The listing builds one solid part. Answer for the finished solid, in the listing's coordinates (mm). Face numbers are marked on the shaded views. A direction names the side the tool comes from. Round coordinates to 2 decimals unless told otherwise and drop trailing zeros. Loops run counter-clockwise (first coordinate to the right, second up) from the corner with the lowest first, then second, coordinate; pieces in that order, holes last. Notation, with made-up numbers: (61.5, -23) -> (101.5, -23) arc R21 ccw to (101.5, -15) -> close; hole circle Ø11 at (11, 4). An arc over 180 degrees is marked (long way). One line per question, with ' | ' between items.
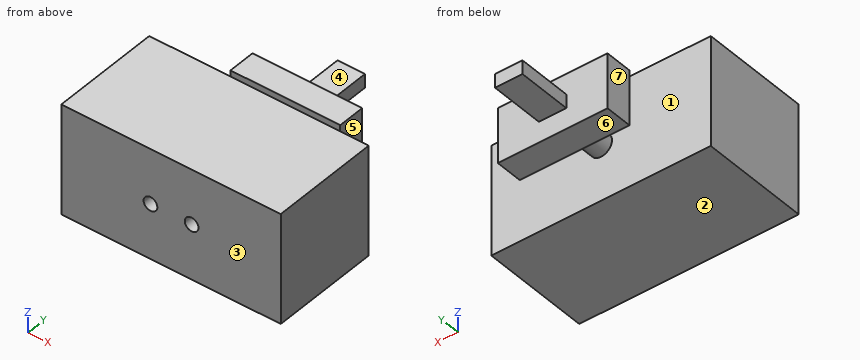
from build123d import *

# Parameters (mm, degrees)
F0_W     = 50.8
F0_H     = 25.4
F0_R     = 1.5875
F1_DEPTH = 25.4
F2_R     = 2.54
F3_DEPTH = 7.62
F4_W     = 25.4
F4_H     = 12.7
F5_DEPTH = 6.35
F6_W     = 6.35
F6_H     = 3.175
F7_DEPTH = 12.7
F8_DEPTH = 19.05


with BuildPart() as f1:
    # F0 (on Front) → F1 (new body)
    with BuildSketch(Plane.XZ):
        Rectangle(F0_W, F0_H)
        with Locations((-4.7625, 0)):
            Circle(F0_R, mode=Mode.SUBTRACT)
        with Locations((4.7625, 0)):
            Circle(F0_R, mode=Mode.SUBTRACT)
        with Locations((4.7625, 0)):
            Circle(F0_R)
        with Locations((-4.7625, 0)):
            Circle(F0_R)
    extrude(amount=-F1_DEPTH)

    # F2 (on face) → F3 (join)
    with BuildSketch(Plane(origin=(0, 25.4, 0), x_dir=(-1, 0, 0), z_dir=(0, 1, 0))):
        Circle(F2_R)
    extrude(amount=F3_DEPTH)

    # F4 (on face) → F5 (join)
    with BuildSketch(Plane(origin=(0, 33.02, 0), x_dir=(-1, 0, 0), z_dir=(0, 1, 0))):
        Rectangle(F4_W, F4_H)
    extrude(amount=F5_DEPTH)

    # F6 (on face) → F7 (join)
    with BuildSketch(Plane(origin=(0, 39.37, 0), x_dir=(-1, 0, 0), z_dir=(0, 1, 0))):
        Rectangle(F6_W, F6_H)
    extrude(amount=F7_DEPTH)

    # F0 (on Front) → F8 (cut)
    with BuildSketch(Plane.XZ):
        with Locations((4.7625, 0)):
            Circle(F0_R)
        with Locations((-4.7625, 0)):
            Circle(F0_R)
    extrude(amount=-F8_DEPTH, mode=Mode.SUBTRACT)


solid = f1.part
Q1. For the marked faces 4, 5, 6 and 7, determine the directions among +Z, -Z, +X, -X, +Y, -Y from which every point of the face is accessible in a straight line to the end or side of a thin tool.
Numbers:
face 4: +Z, +X, -X, +Y | face 5: +Z, -Z, +X, +Y | face 6: -Z, +X, -X, +Y | face 7: +Z, -Z, -X, +Y
Q2. A cutting plane is placed at B-B on x = -11. Give the vertices of the cut face in (y, z), plus the area to 3 significant figures.
Numbers:
outline: (0, -12.7) -> (25.4, -12.7) -> (25.4, 12.7) -> (0, 12.7) -> close; (33.02, -6.35) -> (39.37, -6.35) -> (39.37, 6.35) -> (33.02, 6.35) -> close | area: 726 mm^2
Q3. A cutting plane is placed at C-C on z = 0. Give the vertices of the cut face in (x, y) (3 decimals), plus the area to 3 significant figures.
Numbers:
outline: (-25.4, 0) -> (-6.35, 0) -> (-6.35, 19.05) -> (-3.175, 19.05) -> (-3.175, 0) -> (3.175, 0) -> (3.175, 19.05) -> (6.35, 19.05) -> (6.35, 0) -> (25.4, 0) -> (25.4, 25.4) -> (2.54, 25.4) -> (2.54, 33.02) -> (12.7, 33.02) -> (12.7, 39.37) -> (3.175, 39.37) -> (3.175, 52.07) -> (-3.175, 52.07) -> (-3.175, 39.37) -> (-12.7, 39.37) -> (-12.7, 33.02) -> (-2.54, 33.02) -> (-2.54, 25.4) -> (-25.4, 25.4) -> close | area: 1,450 mm^2
Q4. Find the intervals of material crossed by line 1 (Y direction, x = -9.5, z = 0); line 2 (Y direction, x = -6, z = 0.5); line 3 (X direction, y = 34, z = 0.75), in increasing order. Write a range as from..to.
Numbers:
line 1: 0..25.4, 33.02..39.37 | line 2: 19.05..25.4, 33.02..39.37 | line 3: -12.7..12.7
Q5. For a pull along Y with two mould halves and no side action, classify the marked faces 1, 2 and 3 as pulls with the +Y half, pulls with the -Y half, needs draft (parallel to the pull), parting line crosses it, or undercut.
Numbers:
face 1: undercut | face 2: needs draft | face 3: pulls with the -Y half
Q6. Given pin 1 Ø7.5 at (x, z) = (7, -6) entering from +Y; pin 2 Ø1.9 at (x, y) = (1.5, 37.5) entering from +Z; pin 3 Ø1.6 at (y, z) = (48, 0.5) entering from +X (3 decimals), each flat-ended and moving along its own axis, determine where each tip first touches the part or whether it passes through.
Numbers:
pin 1: y = 39.37 | pin 2: z = 6.35 | pin 3: x = 3.175
Q7. A cutting plane is placed at D-D on x = 0. Give the vertices of the cut face in (y, z), plus the area to 3 significant figures.
Numbers:
outline: (0, -12.7) -> (25.4, -12.7) -> (25.4, -2.54) -> (33.02, -2.54) -> (33.02, -6.35) -> (39.37, -6.35) -> (39.37, -1.59) -> (52.07, -1.59) -> (52.07, 1.59) -> (39.37, 1.59) -> (39.37, 6.35) -> (33.02, 6.35) -> (33.02, 2.54) -> (25.4, 2.54) -> (25.4, 12.7) -> (0, 12.7) -> close | area: 805 mm^2
Q8. A cutting plane is placed at A-A on z = -3.75. Give the vertices of the cut face in (x, y), plus the area to 3 significant figures.
Numbers:
outline: (-25.4, 0) -> (25.4, 0) -> (25.4, 25.4) -> (-25.4, 25.4) -> close; (-12.7, 33.02) -> (12.7, 33.02) -> (12.7, 39.37) -> (-12.7, 39.37) -> close | area: 1,450 mm^2
